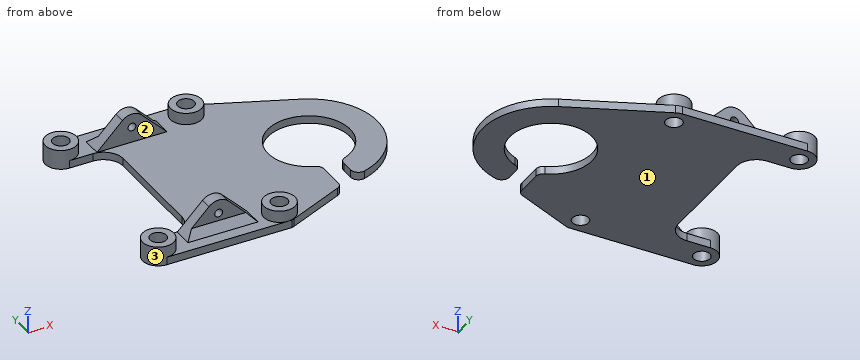
from build123d import *

# Parameters (mm, degrees)
SKETCH1_R                = 2.1
BOSS_EXTRUDE1_DEPTH      = 2
BOSS_EXTRUDE2_START      = -8
SKETCH2_R                = 1
BOSS_EXTRUDE2_DEPTH      = 3
CHAMFER1_SIZE            = 2
CHAMFER1_OF_MIRROR2_SIZE = 2
SKETCH3_R                = 4
SKETCH3_R_2              = 2.1
BOSS_EXTRUDE3_DEPTH      = 3


with BuildPart() as part:
    # Sketch1 → Boss-Extrude1 (new body)
    with BuildSketch(Plane.XY):
        with BuildLine():
            Line((-16, -26.75), (16, -26.75))
            ThreePointArc((16, -26.75), (16.337730018, -26.650061333), (16.665698596, -26.521663849))
            Line((16.665698596, -26.521663849), (31.3079825, -20.055119449))
            ThreePointArc((31.3079825, -20.055119449), (32.175703584, -19.31738929), (32.5, -18.225593751))
            Line((32.5, -18.225593751), (32.5, -11.66190379))
            ThreePointArc((32.5, -11.66190379), (32.14924225, -10.53053294), (31.22, -9.795999183))
            ThreePointArc((31.22, -9.795999183), (35, 10.5), (38.78, -9.795999183))
            ThreePointArc((38.78, -9.795999183), (37.85075775, -10.53053294), (37.5, -11.66190379))
            Line((37.5, -11.66190379), (37.5, -14.832396974))
            ThreePointArc((37.5, -14.832396974), (38.308633206, -16.438835632), (40.080645161, -16.746254648))
            ThreePointArc((40.080645161, -16.746254648), (52.47471331, -0.940422641), (41.848535598, 16.104271488))
            Line((41.848535598, 16.104271488), (17.565379565, 26.43097634))
            ThreePointArc((17.565379565, 26.43097634), (16.798778642, 26.669432699), (16, 26.75))
            Line((16, 26.75), (-16, 26.75))
            ThreePointArc((-16, 26.75), (-20, 22.75), (-16, 18.75))
            Line((-16, 18.75), (-10, 18.75))
            ThreePointArc((-10, 18.75), (-6.464466094, 17.285533906), (-5, 13.75))
            Line((-5, 13.75), (-5, -13.75))
            ThreePointArc((-5, -13.75), (-6.464466094, -17.285533906), (-10, -18.75))
            Line((-10, -18.75), (-16, -18.75))
            ThreePointArc((-16, -18.75), (-20, -22.75), (-16, -26.75))
        make_face()
        with Locations((-16, 22.75)):
            Circle(SKETCH1_R, mode=Mode.SUBTRACT)
        with Locations((16, 22.75)):
            Circle(SKETCH1_R, mode=Mode.SUBTRACT)
        with Locations((15, -22.75)):
            Circle(SKETCH1_R, mode=Mode.SUBTRACT)
        with Locations((-16, -22.75)):
            Circle(SKETCH1_R, mode=Mode.SUBTRACT)
    extrude(amount=BOSS_EXTRUDE1_DEPTH)

    # Sketch2 → Boss-Extrude2 (add)
    with BuildSketch(Plane.XZ.offset(26.75).offset(BOSS_EXTRUDE2_START)):
        with BuildLine():
            Line((-2.474873734, 8.474873734), (-8.949747468, 2))
            Line((-8.949747468, 2), (8.949747468, 2))
            Line((8.949747468, 2), (2.474873734, 8.474873734))
            ThreePointArc((2.474873734, 8.474873734), (0, 9.5), (-2.474873734, 8.474873734))
        make_face()
        with Locations((0, 6)):
            Circle(SKETCH2_R, mode=Mode.SUBTRACT)
    boss_extrude2 = extrude(amount=BOSS_EXTRUDE2_DEPTH)

    # Chamfer1
    chamfer1_edges = [part.edges().sort_by_distance(p)[0] for p in [
        (0, -21.75, 2),
    ]]
    chamfer(chamfer1_edges, length=CHAMFER1_SIZE)

    # Mirror2: Boss-Extrude2 across plane
    add(boss_extrude2.mirror(Plane.ZX))

    # Chamfer1 of Mirror2
    chamfer1_of_mirror2_edges = [part.edges().sort_by_distance(p)[0] for p in [
        (0, 21.75, 2),
    ]]
    chamfer(chamfer1_of_mirror2_edges, length=CHAMFER1_OF_MIRROR2_SIZE)

    # Sketch3 → Boss-Extrude3 (add)
    with BuildSketch(Plane.XY.offset(2)):
        with Locations((-16, -22.75)):
            Circle(SKETCH3_R)
        with Locations((-16, -22.75)):
            Circle(SKETCH3_R_2, mode=Mode.SUBTRACT)
        with Locations((15, -22.75)):
            Circle(SKETCH3_R)
        with Locations((15, -22.75)):
            Circle(SKETCH3_R_2, mode=Mode.SUBTRACT)
        with Locations((16, 22.75)):
            Circle(SKETCH3_R)
        with Locations((16, 22.75)):
            Circle(SKETCH3_R_2, mode=Mode.SUBTRACT)
        with Locations((-16, 22.75)):
            Circle(SKETCH3_R)
        with Locations((-16, 22.75)):
            Circle(SKETCH3_R_2, mode=Mode.SUBTRACT)
    extrude(amount=BOSS_EXTRUDE3_DEPTH)


solid = part.part
Input: part model. Units: mm. Frame: model coordinates. Face numbers are marked on the shaded views. A direction names the side the tool comes from. Give positions to 0.01 mm unless a question says otherwise; leave off trailing zeros. Order: outer loops, then holes, each group sorted by start corner. A loop starts at its lowest first (then second) coordinate and runs counter-clockwise, first axis right, second up. Notation, with made-up numbers: (3.5, -5.75) - (18.5, -5.75) arc R24 cw to (18.5, 27.25) - close; hole circle Ø9 at (-23.75, 39.5). An arc over 180 degrees is marked (long way). Answer as a JSON object with one key per item and string values. Group by question number.
Q1. Line query: probe 1 along Z at (x, y) = (0, -19); probe 2 along X at (y, z) = (0, 1.1); probe 3 along Z at (x, y) = (0.5, 10.5). Output: solid intervals per line, ascending.
Q2. Set-up query: the marked faces 1, 2 and 3. Return all of +Z, -Z, +X, -X, +Y, -Y with unobstructed straight access to the full face (end or side cutting, diameter ignored); none if empty.
Q3. Cut plane A-A, the plane y = 0. Output: boundary loops of the cut face in (x, z).
Q4. Cut plane D-D, the plane z = 6. Output: boundary loops of the cut face in (x, y).
Q5. Cut plane C-C, the plane y = -22.75. Output: boundary loops of the cut face in (x, z), then the cut area to 3 significant figures.
Q6. Cut plane B-B, the plane z = 1.25. Output: boundary loops of the cut face in (x, y), then the cut area to 3 significant figures.
Q7. First-contact query: pin 1 Ø4 at (x, y) = (-15.5, -23) entering from +Z; pin 2 Ø10 at (x, y) = (-8.5, 0) entering from +Z; pin 3 Ø4 at (x, y) = (-3.5, -16.5) entering from -Z; pin 4 Ø1.6 at (y, z) = (-16.5, 1) entering from +X. Flat tips, straight axial feed; report the tip coordinate or a pass-through.
Results:
{
 "1": {"probe 1": "0 to 5, 7 to 9.5", "probe 2": "-5 to 24.5, 45.5 to 52.5", "probe 3": "0 to 2"},
 "2": {"face 1": "-Z, +X, -X, +Y, -Y", "face 2": "+Z, +X, -X", "face 3": "+Z"},
 "3": {"outline": "(-5, 0) - (24.5, 0) - (24.5, 2) - (-5, 2) - close; (45.5, 0) - (52.5, 0) - (52.5, 2) - (45.5, 2) - close"},
 "4": {"outline": "(-4.95, -21.75) - (-1, -21.75) - (-1, -18.75) - (-4.95, -18.75) - close; (-4.95, 18.75) - (-1, 18.75) - (-1, 21.75) - (-4.95, 21.75) - close; (1, -21.75) - (4.95, -21.75) - (4.95, -18.75) - (1, -18.75) - close; (1, 18.75) - (4.95, 18.75) - (4.95, 21.75) - (1, 21.75) - close"},
 "5": {"outline": "(-20, 0) - (-18.1, 0) - (-18.1, 5) - (-20, 5) - close; (-13.9, 0) - (12.9, 0) - (12.9, 5) - (11, 5) - (11, 2) - (8.95, 2) - (7.95, 3) - (-7.95, 3) - (-8.95, 2) - (-12, 2) - (-12, 5) - (-13.9, 5) - close; (17.1, 0) - (25.21, 0) - (25.21, 2) - (19, 2) - (19, 5) - (17.1, 5) - close", "area": "113 mm^2"},
 "6": {"outline": "(-16, -26.75) - (16, -26.75) arc R4.12 ccw to (16.67, -26.52) - (31.31, -20.06) arc R2 ccw to (32.5, -18.23) - (32.5, -11.66) arc R2 ccw to (31.22, -9.8) arc R10.5 cw (long way) to (38.78, -9.8) arc R2 ccw to (37.5, -11.66) - (37.5, -14.83) arc R2 ccw to (40.08, -16.75) arc R17.5 ccw to (41.85, 16.1) - (17.57, 26.43) arc R4 ccw to (16, 26.75) - (-16, 26.75) arc R4 ccw to (-16, 18.75) - (-10, 18.75) arc R5 cw to (-5, 13.75) - (-5, -13.75) arc R5 cw to (-10, -18.75) - (-16, -18.75) arc R4 ccw to start; hole circle Ø4.2 at (-16, -22.75); hole circle Ø4.2 at (-16, 22.75); hole circle Ø4.2 at (15, -22.75); hole circle Ø4.2 at (16, 22.75)", "area": "2,270 mm^2"},
 "7": {"pin 1": "z = 5", "pin 2": "z = 2", "pin 3": "z = 0", "pin 4": "x = 42.73"}
}
